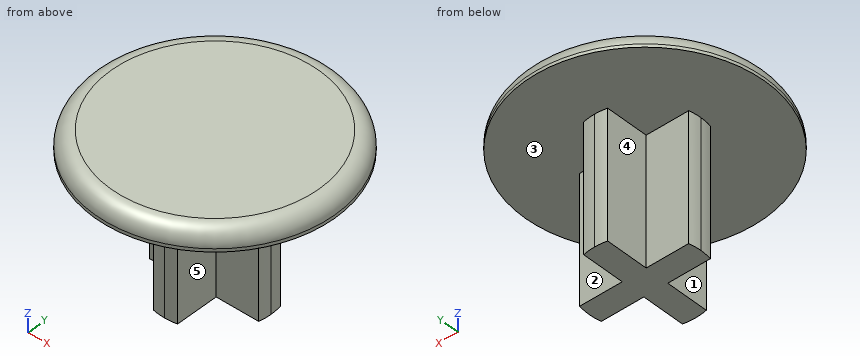
```python
from build123d import *

# Parameters (mm, degrees)
F0_R      = 19.05
F1_DEPTH  = 3.048
F2_R      = 2.54
F3_W      = 17.78
F3_H      = 3.81
F4_W      = 3.81
F4_H      = 6.985
F4_W_2    = 6.985
F4_H_2    = 3.81
F5_DEPTH  = 20.32
F7_DEPTH  = 20.32
F8_DEPTH  = 20.32
F9_DEPTH  = 20.32
F10_DEPTH = 20.32
F11_DEPTH = 20.32


with BuildPart() as f1:
    # F0 (on Top) → F1 (new body)
    with BuildSketch(Plane.XY):
        Circle(F0_R)
    extrude(amount=F1_DEPTH)

    # F2
    f2_edges = [f1.edges().sort_by_distance(p)[0] for p in [
        (-19.05, 0, 3.048),
    ]]
    fillet(f2_edges, radius=F2_R)

    # F3 (on face) + F4 (on face) → F5 (join)
    with BuildSketch(Plane(origin=(0, 0, 0), x_dir=(1, 0, 0), z_dir=(0, 0, -1))):
        Rectangle(F3_W, F3_H)
    with BuildSketch(Plane(origin=(0, 0, 0), x_dir=(1, 0, 0), z_dir=(0, 0, -1))):
        with Locations((0, -5.3975)):
            Rectangle(F4_W, F4_H)
        with Locations((0, 5.3975)):
            Rectangle(F4_W, F4_H)
        with Locations((-5.3975, 0)):
            Rectangle(F4_W_2, F4_H_2)
        with Locations((5.3975, 0)):
            Rectangle(F4_W_2, F4_H_2)
        Rectangle(F4_W, F4_H_2)
    extrude(amount=F5_DEPTH)

    # F6 (on face) → F7 (cut)
    with BuildSketch(Plane(origin=(0, 0, -20.32), x_dir=(1, 0, 0), z_dir=(0, 0, -1))):
        with BuildLine():
            ThreePointArc((0, 8.89), (0.9580800544, 8.8382228196), (1.905, 8.6834944003))
            Line((1.905, 8.6834944003), (1.905, 8.89))
            Line((1.905, 8.89), (0, 8.89))
        make_face()
    extrude(amount=-F7_DEPTH, mode=Mode.SUBTRACT)

    # F6 (on face) → F8 (cut)
    with BuildSketch(Plane(origin=(0, 0, -20.32), x_dir=(1, 0, 0), z_dir=(0, 0, -1))):
        with BuildLine():
            ThreePointArc((-1.905, 8.6834944003), (-0.9580800544, 8.8382228196), (0, 8.89))
            Line((0, 8.89), (-1.905, 8.89))
            Line((-1.905, 8.89), (-1.905, 8.6834944003))
        make_face()
    extrude(amount=-F8_DEPTH, mode=Mode.SUBTRACT)

    # F6 (on face) → F9 (cut)
    with BuildSketch(Plane(origin=(0, 0, -20.32), x_dir=(1, 0, 0), z_dir=(0, 0, -1))):
        with BuildLine():
            Line((-8.89, -1.905), (-8.6834944003, -1.905))
            ThreePointArc((-8.6834944003, -1.905), (-8.8382228196, -0.9580800544), (-8.89, 0))
            Line((-8.89, 0), (-8.89, -1.905))
        make_face()
    extrude(amount=-F9_DEPTH, mode=Mode.SUBTRACT)

    # F6 (on face) → F10 (cut)
    with BuildSketch(Plane(origin=(0, 0, -20.32), x_dir=(1, 0, 0), z_dir=(0, 0, -1))):
        with BuildLine():
            ThreePointArc((-8.89, 0), (-8.8382228196, 0.9580800544), (-8.6834944003, 1.905))
            Line((-8.6834944003, 1.905), (-8.89, 1.905))
            Line((-8.89, 1.905), (-8.89, 0))
        make_face()
    extrude(amount=-F10_DEPTH, mode=Mode.SUBTRACT)

    # F6 (on face) → F11 (cut)
    with BuildSketch(Plane(origin=(0, 0, -20.32), x_dir=(1, 0, 0), z_dir=(0, 0, -1))):
        with BuildLine():
            Line((1.905, -8.89), (1.905, -8.6834944003))
            ThreePointArc((1.905, -8.6834944003), (0.9580800544, -8.8382228196), (0, -8.89))
            Line((0, -8.89), (1.905, -8.89))
        make_face()
        with BuildLine():
            Line((-1.905, -8.89), (0, -8.89))
            ThreePointArc((0, -8.89), (-0.9580800544, -8.8382228196), (-1.905, -8.6834944003))
            Line((-1.905, -8.6834944003), (-1.905, -8.89))
        make_face()
        with BuildLine():
            Line((8.89, -1.905), (8.89, 0))
            ThreePointArc((8.89, 0), (8.8382228196, -0.9580800544), (8.6834944003, -1.905))
            Line((8.6834944003, -1.905), (8.89, -1.905))
        make_face()
        with BuildLine():
            ThreePointArc((8.6834944003, 1.905), (8.8382228196, 0.9580800544), (8.89, 0))
            Line((8.89, 0), (8.89, 1.905))
            Line((8.89, 1.905), (8.6834944003, 1.905))
        make_face()
    extrude(amount=-F11_DEPTH, mode=Mode.SUBTRACT)


solid = f1.part
```
Geometry: final body of the model. Coordinates: model frame, mm. Face numbers are marked on the shaded views. A direction names the side the tool comes from. Coordinates: 2 decimals unless noted, no trailing zeros. Loops run counter-clockwise (first coordinate to the right, second up) from the corner with the lowest first, then second, coordinate; pieces in that order, holes last. Notation, with made-up numbers: M 35.5,55.5 L 52.5,55.5 A23 cw 52.5,66.5 Z; hole C 14.5,67.25 d4. An arc over 180 degrees is marked long. Put each result on its own line as item: value.
(1) Cut plane A-A on z = -12. Return the cut outline in (x, y) (1 decimal), then the cut area to 3 significant figures.
Answer sheet:
outline: M -8.7,-1.9 L -1.9,-1.9 L -1.9,-8.7 A8.9 ccw 1.9,-8.7 L 1.9,-1.9 L 8.7,-1.9 A8.9 ccw 8.7,1.9 L 1.9,1.9 L 1.9,8.7 A8.9 ccw -1.9,8.7 L -1.9,1.9 L -8.7,1.9 A8.9 ccw Z
area: 120 mm^2
(2) Access query for the marked faces 1, 2, 3, 4 and 5. Directions: +Z, -Z, +X, -X, +Y, -Y. A direction counts if a zero-diameter tool reaches every point of the face in a straight line with its end or side. Return the directions, or none.
Answer sheet:
face 1: -Z, -X, -Y
face 2: -Z, +X, +Y
face 3: -Z
face 4: -Z, -X, +Y
face 5: -Z, +X, -Y
(3) First-contact query: pin 1 (7.5 mm diameter, centred on y = -3.5, z = -6, fed in from -X); pin 2 (7.5 mm diameter, centred on x = 3.5, z = -7, fed in from +Y); pin 3 (3 mm diameter, centred on x = -8, z = -1, fed in from -Y). Flat tips, straight axial feed; report the tip coordinate or a pass-through.
Answer sheet:
pin 1: stops at x = -8.89
pin 2: stops at y = 8.89
pin 3: stops at y = -17.76
(4) Material intervals for probe 1 along Y at (x, z) = (7.5, -13.5) (3 decimals); probe 2 along Z at (x, y) = (-4, -9.5), sorted ascending.
Answer sheet:
probe 1: y = -1.905 to 1.905
probe 2: z = 0 to 3.05
